```python
from build123d import *

# Parameters (mm, degrees)
F0_R          = 5.1
F0_R_2        = 6.1
F1_DEPTH      = 34.5
F2_R          = 4
F3_T          = 4
F4_DEPTH      = 50
F4_DEPTH_BACK = 50
F5_R          = 3
F7_D          = 11
F9_D          = 6.8


# Not quite as in the source:
# - ends of sketch curves that miss each other by under 0.0002 mm in the source are joined
# - a shell that OpenCascade refuses in one call is made with other operations: the cavity is built on its own and cut out
# - a feature names something its author has since deleted; it is built from what else it names


with BuildPart() as f1:
    # F0 (on Right) → F1 (new body, symmetric)
    with BuildSketch(Plane.YZ):
        with BuildLine():
            Line((1.885386, -78.484767), (45, -78.484767))
            Line((45, -78.484767), (28.944748, -25.970405))
            Line((28.944748, -25.970405), (33.917533, -24.450072))
            Line((33.917533, -24.450072), (13.451514, 42.49126))
            Line((13.451514, 42.49126), (8.478729, 40.970928))
            Line((8.478729, 40.970928), (-0.714257, 71.03983))
            ThreePointArc((-0.714257, 71.03983), (-21.6924256797, 84.2760694236), (-37.884047, 65.484768))
            Line((-37.884047, 65.484768), (-37.884047, -78.484767))
            Line((-37.884047, -78.484767), (-3.771468, -78.484767))
            Line((-3.771468, -78.484767), (1.885386, -78.484767))
        make_face()
        with Locations((-18.884047, -44.984767)):
            Circle(F0_R, mode=Mode.SUBTRACT)
        with Locations((-18.893362, 65.515233)):
            Circle(F0_R_2, mode=Mode.SUBTRACT)
    extrude(amount=F1_DEPTH, both=True)

    # F2
    f2_edges = [f1.edges().sort_by_distance(p)[0] for p in [
        (-34.5, 23.684523, 9.020594),
        (34.5, 23.684523, 9.020594),
    ]]
    fillet(f2_edges, radius=F2_R)

    # F3: shell of thickness 4, made by hand


with BuildPart() as f3_core1:
    # F3_t2: copy of F1
    add(f1.part)

    # the walls: a layer under each face that stays
    f3_faces = [f3_core1.faces().sort_by_distance(p)[0] for p in [
        (-34.5, 3.5579765, 3.0000004813),
        (0, 23.6845235, 9.020594),
        (34.5, 3.5579765, 3.0000004813),
    ]]
    thicken(f3_faces, amount=-F3_T, mode=Mode.SUBTRACT)


with BuildPart() as f1_1:
    add(f1.part)

    # what is left inside the walls is the cavity
    f3_cavity = [f3_core1.part.solids().sort_by_distance(p)[0] for p in [
        (-30.46, 3.557976, -24.161589),
    ]]
    add(f3_cavity, mode=Mode.SUBTRACT)

    # F0 (on Right) → F4 (join, two sides)
    with BuildSketch(Plane.YZ) as f4_sk:
        Polygon((-105, -84.484767), (105, -84.484767), (105, -78.484767), (45, -78.484767), (1.885386, -78.484767), (-3.771468, -78.484767), (-37.884047, -78.484767), (-105, -78.484767), align=None)
    extrude(amount=F4_DEPTH)
    extrude(f4_sk.sketch, amount=-F4_DEPTH_BACK)

    # F5
    f5_edges = [f1_1.edges().sort_by_distance(p)[0] for p in [
        (-50, -105, -81.484767),
        (50, -105, -81.484767),
        (50, 105, -81.484767),
        (-50, 105, -81.484767),
    ]]
    fillet(f5_edges, radius=F5_R)

    # F7 (through all)
    with Locations(Plane.XY.offset(-78.484767)):
        with Locations((-35, 90), (-35, -90), (35, -90), (35, 90)):
            Hole(F7_D / 2)

    # F9 (through all)
    with Locations(Plane(origin=(0, 24.1820677637, 7.3932000384), x_dir=(-1, 0, 0), z_dir=(0, 0.9563047562, 0.2923717041))):
        with Locations((0, 22.7017519629), (0, -19.2982480371)):
            Hole(F9_D / 2)


solid = f1_1.part
```
Verification items for the finished model (mm, model axes). A direction names the side the tool comes from. Coordinates: 2 decimals unless noted, no trailing zeros. Order: outer loops, then holes, each group sorted by start corner. A loop starts at its lowest first (then second) coordinate and runs counter-clockwise, first axis right, second up. Notation, with made-up numbers: (49.25, 57) - (63.25, 57) arc R10 cw to (63.25, 63) - close; hole circle Ø10 at (-39, 37.25). An arc over 180 degrees is marked (long way). Return JSON: item names as keys, results as strings.
(1) Thickness scan on line 1 along Y through (x, z) = (35, -82); line 2 along X through (y, z) = (-20, -25); line 3 along Z through (x, y) = (-29.5, -43.5). Record the ranges inside material, lowest first.
Filled sheet:
{"line 1": "y = -105 to -95.5, -84.5 to 84.5, 95.5 to 105", "line 2": "x = -34.5 to -30.5, 30.5 to 34.5", "line 3": "z = -84.48 to -78.48"}
(2) Section check C-C, the plane y = -35. Record the cut outline in (x, z).
Filled sheet:
{"outline": "(-50, -84.48) - (50, -84.48) - (50, -78.48) - (34.5, -78.48) - (34.5, 75.55) - (30.5, 75.55) - (30.5, -78.48) - (-30.5, -78.48) - (-30.5, 75.55) - (-34.5, 75.55) - (-34.5, -78.48) - (-50, -78.48) - close"}
(3) Section check B-B, the plane y = -90. Record the cut outline in (x, z), and give its area (3 significant figures).
Filled sheet:
{"outline": "(-50, -84.48) - (-40.5, -84.48) - (-40.5, -78.48) - (-50, -78.48) - close; (-29.5, -84.48) - (29.5, -84.48) - (29.5, -78.48) - (-29.5, -78.48) - close; (40.5, -84.48) - (50, -84.48) - (50, -78.48) - (40.5, -78.48) - close", "area": "468 mm^2"}
(4) Go/stop test with flat-tipped pins: pin 1 (1.5 mm diameter, centred on x = -9, z = -5.5, fed in from -Y); pin 2 (2 mm diameter, centred on x = -32.5, z = -30, fed in from -Y); pin 3 (16 mm diameter, centred on y = -18.89, z = 65.52, fed in from -X); pin 4 (6 mm diameter, centred on y = -18.88, z = -44.98, fed in from +X). Record where each tip stops, or that it passes through.
Filled sheet:
{"pin 1": "stops at y = 23.71", "pin 2": "stops at y = -37.88", "pin 3": "stops at x = -34.5", "pin 4": "passes through"}
(5) Section check A-A, the plane x = 19.5. Record the cut outline in (y, z).
Filled sheet:
{"outline": "(-105, -84.48) - (105, -84.48) - (105, -78.48) - (-105, -78.48) - close; (9.63, 41.32) - (30.09, -25.62) - (33.92, -24.45) - (13.45, 42.49) - close"}
(6) Mould release check, pull along X, two halves, no side actions. Record for faces 4 (the cylindrical face through (32.47, -22.93, -48.09)), 5 (the flat face through (50, -1, -81)), 6 (the flat face through (0.427, 20.003, 7.383)): pulls with the +X half, pulls with the -X half, needs draft (parallel to the pull), parting line crosses it, or undercut.
Filled sheet:
{"face 4": "needs draft", "face 5": "pulls with the +X half", "face 6": "undercut"}
(7) Access from +Z, -Z, +X, -X, +Y, -Y to the whole of each face (thin tool, end or side, straight path). Record for faces 1 (the flat face through (32.528, 37.085, -52.595)), 2 (the cylindrical face through (-0.44, 26.9, -8.43)), 3 (the flat face through (30.5, -6, -14)).
Filled sheet:
{"face 1": "+X, -X, +Y", "face 2": "none", "face 3": "-Y"}
